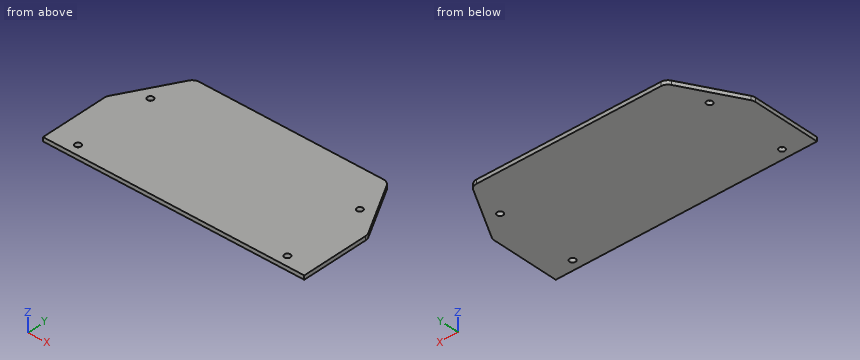
from build123d import *

# Parameters (mm, degrees)
ESQUISSE1_R               = 1.5
T_LE_DE_BASE_PLI_E1_DEPTH = 2
CONG_1_R                  = 4


# Sheet-metal steps are written as plain solids
with BuildPart() as part:
    # Esquisse1 → Tôle de base pliée1 (new body)
    with BuildSketch(Plane.XY):
        Polygon((-48.526816654, 65), (-65.5, 35), (-65.5, 0), (65.5, 0), (65.5, 35), (48.526816654, 65), align=None)
        with Locations((-52.5, 45)):
            Circle(ESQUISSE1_R, mode=Mode.SUBTRACT)
        with Locations((-52.5, 5)):
            Circle(ESQUISSE1_R, mode=Mode.SUBTRACT)
        with Locations(Location((52.5, 5, 0), (0, 0, 180))):
            Circle(ESQUISSE1_R, mode=Mode.SUBTRACT)
        with Locations(Location((52.5, 45, 0), (0, 0, 180))):
            Circle(ESQUISSE1_R, mode=Mode.SUBTRACT)
    extrude(amount=-T_LE_DE_BASE_PLI_E1_DEPTH)

    # Congé1
    cong_1_edges = [part.edges().sort_by_distance(p)[0] for p in [
        (-65.5, 35, -1),
        (-48.526816654, 65, -1),
        (48.526816654, 65, -1),
        (65.5, 35, -1),
    ]]
    fillet(cong_1_edges, radius=CONG_1_R)


solid = part.part
Design review of the part built by this model. Coordinates are the model's own, in mm. Coordinates: 2 decimals unless noted, no trailing zeros. Order: outer loops, then holes, each group sorted by start corner. A loop starts at its lowest first (then second) coordinate and runs counter-clockwise, first axis right, second up.
Item 1: For pin 1 Ø12 at (x, y) = (-4.5, 28.5) entering from +Z; pin 2 Ø1.8 at (x, y) = (52.5, 45) entering from -Z, all flat-tipped, find the tip position at first contact; note any pin that passes through.
Item 2: For line 1 (Y direction, x = -52.5, z = -1.4); line 2 (Y direction, x = -53.5, z = -1.3); line 3 (X direction, y = 61, z = -1.4), list the stretches that pass through material, from the lowest coordinate up.
Item 3: Take a section at B-B, the plane z = -1.7. Write out the cut boundary in (x, y), then the cut area to 3 significant figures.
Item 4: Take a section at D-D, the plane y = 38.5. Write out the cut boundary in (x, z).
Item 5: Take a section at A-A, the plane y = 5. Write out the cut boundary in (x, z).
Item 6: Take a section at C-C, the plane x = -52.5. Write out the cut boundary in (y, z).
The answers:
1. pin 1: stops at z = 0
1. pin 2: passes through
2. line 1: y = 0 to 3.5, 6.5 to 43.5, 46.5 to 57.98
2. line 2: y = 0 to 3.88, 6.12 to 43.88, 46.12 to 56.21
2. line 3: x = -50.79 to 50.79
3. outline: (-65.5, 0) - (65.5, 0) - (65.5, 33.95) arc R4 ccw to (64.98, 35.92) - (49.68, 62.97) arc R4 ccw to (46.19, 65) - (-46.19, 65) arc R4 ccw to (-49.68, 62.97) - (-64.98, 35.92) arc R4 ccw to (-65.5, 33.95) - close; hole circle Ø3 at (-52.5, 5); hole circle Ø3 at (-52.5, 45); hole circle Ø3 at (52.5, 5); hole circle Ø3 at (52.5, 45)
3. area: 7,980 mm2
4. outline: (-63.52, -2) - (63.52, -2) - (63.52, 0) - (-63.52, 0) - close
5. outline: (-65.5, -2) - (-54, -2) - (-54, 0) - (-65.5, 0) - close; (-51, -2) - (51, -2) - (51, 0) - (-51, 0) - close; (54, -2) - (65.5, -2) - (65.5, 0) - (54, 0) - close
6. outline: (0, -2) - (3.5, -2) - (3.5, 0) - (0, 0) - close; (6.5, -2) - (43.5, -2) - (43.5, 0) - (6.5, 0) - close; (46.5, -2) - (57.98, -2) - (57.98, 0) - (46.5, 0) - close
